from build123d import *

# Parameters (mm, degrees)
BOSS_EXTRUDE1_DEPTH = 1143
Y_FACE_DEPTH        = 39.1
X_FACE_DEPTH        = 39.1


with BuildPart() as part:
    # Sketch2 → Boss-Extrude1 (new body)
    with BuildSketch(Plane.XY):
        Polygon((0, 0), (0, -38.1), (6.35, -38.1), (6.35, -6.35), (38.1, -6.35), (38.1, 0), align=None)
    extrude(amount=BOSS_EXTRUDE1_DEPTH)

    # Sketch3 → Y Face (cut, through all)
    with BuildSketch(Plane(origin=(0, 0, 0), x_dir=(1, 0, 0), z_dir=(0, 1, 0))):
        Polygon((6.35, 0), (6.35, -31.75), (38.1, -43.790982062), (38.1, 0), align=None)
        Polygon((38.1, -1046.772380605), (0, -1143), (38.1, -1143), align=None)
    extrude(amount=-Y_FACE_DEPTH, mode=Mode.SUBTRACT)

    # Sketch4 → X Face (cut, through all)
    with BuildSketch(Plane.ZY):
        Polygon((1143, 0), (1135.00664554, -38.1), (1143, -38.1), align=None)
        Polygon((0, -38.1), (21.672171987, -38.1), (29.665526448, 0), (0, 0), align=None)
    extrude(amount=-X_FACE_DEPTH, mode=Mode.SUBTRACT)


solid = part.part
Can you work these out from the model? Positions are in its coordinate system, mm. Give positions to 0.01 mm unless a question says otherwise; leave off trailing zeros. Loops run counter-clockwise (first coordinate to the right, second up) from the corner with the lowest first, then second, coordinate; pieces in that order, holes last. Notation, with made-up numbers: M 84.25,69 L 111.25,69 A25 cw 111.25,85 Z; hole C 51,-22 d5. An arc over 180 degrees is marked long. One line per item, written item: value. Start each with the question number.
1) If we section it at B-B, the plane y = -13: Write out the boundary of the cut face in (x, z).
2) I'm going to push a flat-ended pin straight in: pin 1 (1.5 mm diameter, centred on y = -17.5, z = 204, fed in from +X). Where does the tip first touch, or does it pass through?
3) If we section it at A-A, the plane z = 94.5: Write out the boundary of the cut face in (x, y), and give its area (3 significant figures).
4) If we section it at C-C, the plane x = 13: Write out the boundary of the cut face in (y, z), and give its area (3 significant figures).
5) If I drill on line 1 (Y direction, x = 20, z = 357); line 2 (X direction, y = -22, z = 682), over which ranges is the centre line in solid material (lowest first)? Write a range as [from, to].
6) Thinking about a two-plate mould opening in Y: for faces 1 (the face through (19, 0, 579)), 2 (the face through (6.35, -23, 567)), 3 (the face through (22, -6.35, 572)), which applies, +Y half, -Y half, draft (parallel to the pull), parting line (faces both ways), or undercut?
Completed:
1. outline: M 0,26.94 L 6.35,26.94 L 6.35,1126.96 L 1.08,1140.27 L 0,1140.27 Z
2. pin 1: stops at x = 6.35
3. outline: M 0,-38.1 L 6.35,-38.1 L 6.35,-6.35 L 38.1,-6.35 L 38.1,0 L 0,0 Z
3. area: 444 mm^2
4. outline: M -6.35,34.27 L 0,34.27 L 0,1110.17 L -6.35,1110.17 Z
4. area: 6,830 mm^2
5. line 1: y = [-6.35, 0]
5. line 2: x = [0, 6.35]
6. face 1: +Y half
6. face 2: draft
6. face 3: -Y half
